Input: part model. Units: mm. Frame: model coordinates. A direction names the side the tool comes from. Coordinates: 2 decimals unless noted, no trailing zeros. Write each loop counter-clockwise with the first axis right and the second up, starting at its lowest first coordinate (ties: lowest second). Pieces come first, ordered by that corner, then holes. Notation, with made-up numbers: (80, 43) - (124, 43) arc R31 ccw to (124, 82) - close; hole circle Ø6 at (40.25, 58). An arc over 180 degrees is marked (long way). Use CSV: the item, a comma, the result in double quotes.
```python
from build123d import *

# Parameters (mm, degrees)
F0_R     = 95
F0_R_2   = 75
F1_DEPTH = 1
F2_DEPTH = 3
F3_D     = 1


with BuildPart() as f1:
    # F0 (on Top) → F1 (new body)
    with BuildSketch(Plane.XY):
        Circle(F0_R)
        Circle(F0_R_2, mode=Mode.SUBTRACT)
        Circle(F0_R_2)
    extrude(amount=F1_DEPTH)

    # F0 (on Top) → F2 (join)
    with BuildSketch(Plane.XY):
        Circle(F0_R_2)
    extrude(amount=F2_DEPTH)

    # F3 (through all)
    with Locations(Plane(origin=(0, 0, 0), x_dir=(1, 0, 0), z_dir=(0, 0, -1))):
        with Locations((0, -75), (-64.9519052838, 37.5), (64.9519052838, 37.5), (82.2724133595, 47.5), (-82.2724133595, 47.5), (0, -95)):
            Hole(F3_D / 2)


solid = f1.part
```
(1) Cut plane C-C on z = 2.15. Return loops of the section in (x, y).
Check values:
outline,"(-65.2, -37.07) arc R0.5 cw to (-64.7, -37.93) arc R75 ccw to (64.7, -37.93) arc R0.5 cw to (65.2, -37.07) arc R75 ccw to (0.5, 75) arc R0.5 cw to (-0.5, 75) arc R75 ccw to start"
(2) Cut plane D-D on y = 79.5. Return loops of the section in (x, z), and give its area (3 significant figures).
Check values:
outline,"(-52.01, 0) - (52.01, 0) - (52.01, 1) - (-52.01, 1) - close"
area,"104 mm^2"
(3) Cut plane B-B on x = -58.5. Return loops of the section in (y, z), and give its area (3 significant figures).
Check values:
outline,"(-74.85, 0) - (74.85, 0) - (74.85, 1) - (46.93, 1) - (46.93, 3) - (-46.93, 3) - (-46.93, 1) - (-74.85, 1) - close"
area,"337 mm^2"
(4) Ray query, probe 1 along Y at (x, z) = (0, 0.6); probe 2 along Z at (x, y) = (82.5, 42.5); probe 3 along X at (y, z) = (-37.5, 0.85). Return the intervals inside material, ascending. Write a range as from..to.
Check values:
probe 1,"-95..74.5, 75.5..94.5"
probe 2,"0..1"
probe 3,"-87.29..-65.45, -64.45..64.45, 65.45..87.29"
(5) Cut plane A-A on y = 47.5. Return loops of the section in (x, z), and give its area (3 significant figures).
Check values:
outline,"(-82.27, 0) - (82.27, 0) - (82.27, 1) - (58.04, 1) - (58.04, 3) - (-58.04, 3) - (-58.04, 1) - (-82.27, 1) - close"
area,"397 mm^2"
(6) Reachability of faces 1 (the cylindrical face through (65.49, 36.55, 1.99)), 2 (the cylindrical face through (-1.093, -74.992, 1.986)), 3 (the flat face through (70, 29, 1)) from +Z, -Z, +X, -X, +Y, -Y: full face, straight path, thin tool, end or side. Return the list, or none.
Check values:
face 1,"+Z, +X"
face 2,"+Z, -Y"
face 3,"+Z"
(7) Pin query (flat end, axial travel): pin 1 Ø1.5 at (y, z) = (-71.5, 0.5) entering from -X. Return the tip coordinate at first contact, or that it passes through.
Check values:
pin 1,"x = -63.4"
